from build123d import *

# Parameters (mm, degrees)
SKETCH1_R           = 1.5
BOSS_EXTRUDE1_DEPTH = 3
SKETCH4_W           = 3.5
SKETCH4_H           = 12
BOSS_EXTRUDE3_DEPTH = 10.5
SKETCH5_W           = 2
SKETCH5_H           = 12
BOSS_EXTRUDE4_DEPTH = 1.1
SKETCH6_W           = 0.2
SKETCH6_H           = 3
BOSS_EXTRUDE5_DEPTH = 0.5
CHAMFER1_SIZE       = 4


with BuildPart() as part:
    # Sketch1 → Boss-Extrude1 (new body)
    with BuildSketch(Plane(origin=(0, 0, 0), x_dir=(1, 0, 0), z_dir=(0, 1, 0))):
        with BuildLine():
            Line((-49, 6), (49, 6))
            ThreePointArc((49, 6), (55, 0), (49, -6))
            Line((49, -6), (-49, -6))
            ThreePointArc((-49, -6), (-55, 0), (-49, 6))
        make_face()
        with Locations(Location((-51.5, 0, 0), (0, 0, 270))):
            Circle(SKETCH1_R, mode=Mode.SUBTRACT)
        with Locations(Location((51.5, 0, 0), (0, 0, 270))):
            Circle(SKETCH1_R, mode=Mode.SUBTRACT)
    extrude(amount=BOSS_EXTRUDE1_DEPTH)

    # Sketch4 → Boss-Extrude3 (add)
    with BuildSketch(Plane.XZ):
        with Locations((-21.690023983, 0)):
            Rectangle(SKETCH4_W, SKETCH4_H)
        with Locations((21.690023983, 0)):
            Rectangle(SKETCH4_W, SKETCH4_H)
    extrude(amount=BOSS_EXTRUDE3_DEPTH)

    # Sketch5 → Boss-Extrude4 (add)
    with BuildSketch(Plane.XZ):
        with Locations((5, 0)):
            Rectangle(SKETCH5_W, SKETCH5_H)
        Rectangle(SKETCH5_W, SKETCH5_H)
        with Locations((10, 0)):
            Rectangle(SKETCH5_W, SKETCH5_H)
        with Locations((-5, 0)):
            Rectangle(SKETCH5_W, SKETCH5_H)
        with Locations((-10, 0)):
            Rectangle(SKETCH5_W, SKETCH5_H)
    extrude(amount=BOSS_EXTRUDE4_DEPTH)

    # Sketch6 → Boss-Extrude5 (add)
    with BuildSketch(Plane.XY.offset(6)):
        with Locations((48.9, 1.5)):
            Rectangle(SKETCH6_W, SKETCH6_H)
        with Locations((-48.9, 1.5)):
            Rectangle(SKETCH6_W, SKETCH6_H)
    extrude(amount=BOSS_EXTRUDE5_DEPTH)

    # Chamfer1
    chamfer1_edges = [part.edges().sort_by_distance(p)[0] for p in [
        (-23.440023983, 0, 0),
        (23.440023983, 0, 0),
    ]]
    chamfer(chamfer1_edges, length=CHAMFER1_SIZE)


solid = part.part
Part model, mm, in its own coordinate system. A direction names the side the tool comes from. Coordinates: 2 decimals unless noted, no trailing zeros. Order: outer loops, then holes, each group sorted by start corner. A loop starts at its lowest first (then second) coordinate and runs counter-clockwise, first axis right, second up. Notation, with made-up numbers: (12, 45.5) - (63, 45.5) arc R24 cw to (63, 79.5) - close; hole circle Ø5 at (35, -22.75). An arc over 180 degrees is marked (long way). Use CSV: the item, a comma, the result in double quotes.
Item 1: Drop flat-ended pins along their axis: P1, Ø0.6, axis at y = 1.5, z = 6.5, coming from the +X side; P2, Ø2, axis at x = -10, z = 0, coming from the -Y side; P3, Ø8, axis at x = 23, y = -0.5, coming from the +Z side; P4, Ø2, axis at x = -17.5, y = -6, coming from the +Z side. Give the stop position or say it passes through.
Solved:
P1,"stops at x = 49"
P2,"stops at y = -1.1"
P3,"stops at z = 6"
P4,"passes through"
Item 2: 3-axis set-ups, long thin cutter, end or side, ignore diameter. For faces 1 (the face through (-22, -10.5, 0)), 2 (the face through (-0.7, -0.8, -6)), 3 (the face through (-2, 0, 0)), 4 (the face through (-41, 0, 0)), 5 (the face through (41, 0, 0)): which of +Z, -Z, +X, -X, +Y, -Y reach the whole face in a straight line?
Solved:
face 1,"+Z, -Z, +X, -X, -Y"
face 2,"-Z, +X, -X, +Y, -Y"
face 3,"+Z, -Z, -Y"
face 4,"+Z, -Z, -X, -Y"
face 5,"+Z, -Z, +X, -Y"
Item 3: Saw through at A-A on y = -8.25. Give the cut face in (x, z), and give its area (3 significant figures).
Solved:
outline,"(-23.44, -6) - (-19.94, -6) - (-19.94, 6) - (-23.44, 6) - close; (19.94, -6) - (23.44, -6) - (23.44, 6) - (19.94, 6) - close"
area,"84.0 mm²"
Item 4: Probe probe 1 along X at (y, z) = (-4, -1.5); probe 2 along X at (y, z) = (-1.25, -1); probe 3 along Y at (x, z) = (46, 3.25). List the from-to ranges inside material, lowest first.
Solved:
probe 1,"x = -23.44 to -19.94, 19.94 to 23.44"
probe 2,"x = -26.19 to -19.94, 19.94 to 26.19"
probe 3,"y = 0 to 3"
Item 5: Mould opens along Z. For faces 6 (the face through (50, 1, 0)), 7 (the face through (-23.44, -7, 0)), 8 (the face through (0.7, -0.8, 6)) say: +Z half, -Z half, draft (parallel to the pull), parting line (faces both ways), or undercut.
Solved:
face 6,"undercut"
face 7,"draft"
face 8,"+Z half"
Item 6: Saw through at B-B on z = 0. Give the number of separate pieces and of enclosed holes in the cut face, and give its area (4 significant figures).
Solved:
separate pieces,"3"
enclosed holes,"0"
area,"412.5 mm²"
Item 7: Saw through at C-C on x = 51.5. Give the cut face in (y, z), and give its area (3 significant figures).
Solved:
outline,"(0, -5.45) - (3, -5.45) - (3, -1.5) - (0, -1.5) - close; (0, 1.5) - (3, 1.5) - (3, 5.45) - (0, 5.45) - close"
area,"23.7 mm²"
